Can you work these out from the drawing? Everything is in mm from the part's minimum corner. A direction names the side the tool comes from. Give positions to 0.01 mm unless a question says otherwise; leave off trailing zeros. Loops run counter-clockwise (first coordinate to the right, second up) from the corner with the lowest first, then second, coordinate; pieces in that order, holes last. Notation, with made-up numbers: (69, 71) - (128, 71) arc R20 cw to (128, 102) - close; hole circle Ø3 at (7.25, 51.5). An arc over 180 degrees is marked (long way). One line per item, written item: value. Start each with the question number.
Q1. For the marked faces 5, 6 and 7, which set-ups out of +Z, -Z, +X, -X, +Y, -Y let a thin tool reach every point of the face, with its end or its side?
Q2. If I drill on line 1 (Z direction, x = 33, y = 20); line 2 (Z direction, x = 6.5, y = 22.5); line 3 (X direction, y = 30, z = 86), over which ranges is the centre line in solid material (lowest first)? Write a range as from..to.
Q3. I want a section at D-D (y = 36). Please give me the cut outline in (x, z), then the cut area to 3 significant figures.
Q4. I want a section at B-B (y = 11.5). Please give me the cut outline in (x, z).
Q5. If we mould it in two halves opening along Z, with no side actions, what happens to the marked faces 1, 2, 3 and 4? For each: released by +Z, released by -Z, zero draft, split by the parting line, or undercut.
Q6. I'm going to push flat-ended pins straight in: P1, Ø23, axis at y = 20, z = 20, coming from the +X side; P2, Ø1.5, axis at x = 30.5, y = 35.5, coming from the +Z side; P3, Ø16, axis at y = 20, z = 100, coming from the +X side; P4, Ø10, axis at x = 17.5, y = 17.5, coming from the -Z side. Where does each tip first touch, or does it pass through?
Q7. I want a section at C-C (x = 8). Count the separate pieces of the cut face and the enclosed holes in it, then the cut area to 3 significant figures.
Q8. I want a section at A-A (z = 35.5). Please give me the cut outline in (x, y).
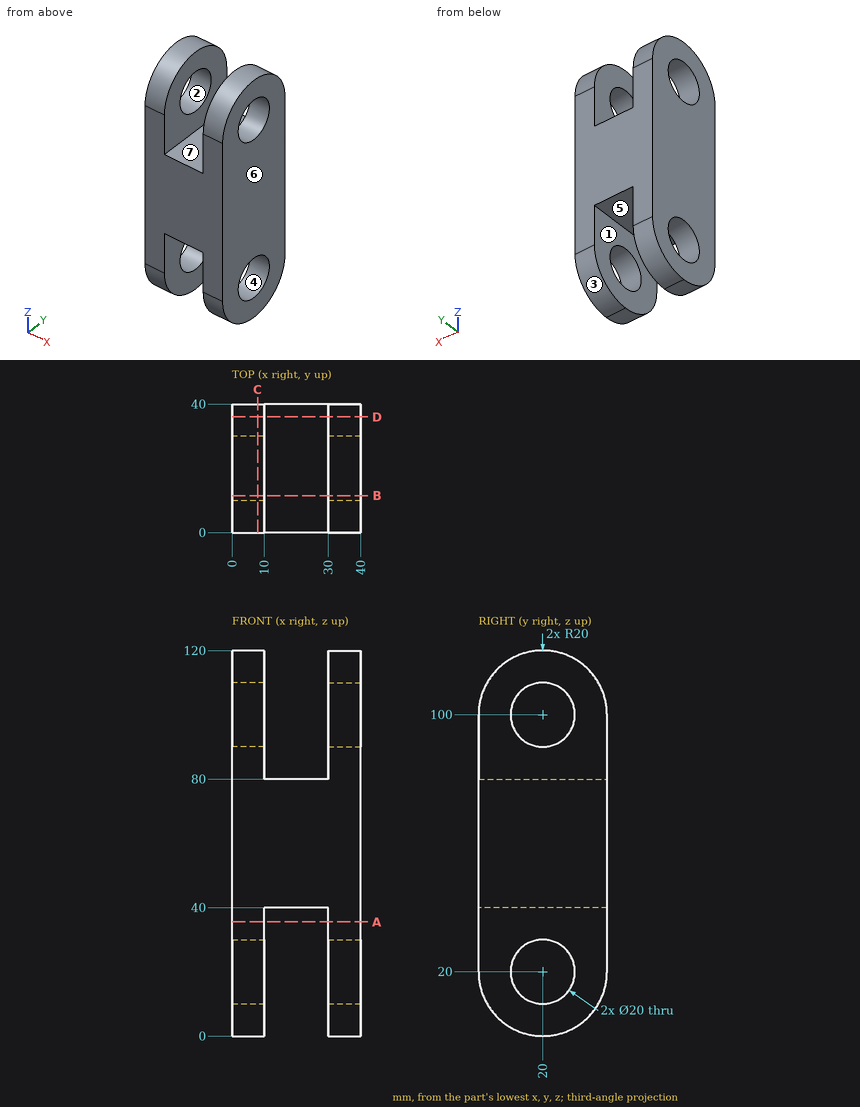
Worked answers:
1. face 5: -Z, +Y, -Y
1. face 6: +Z, -Z, +X, +Y, -Y
1. face 7: +Z, +Y, -Y
2. line 1: z = 0..10, 30..90, 110..120
2. line 2: z = 0.16..10.32, 29.68..90.32, 109.68..119.84
2. line 3: x = 0..10, 30..40
3. outline: (0, 8) - (10, 8) - (10, 40) - (30, 40) - (30, 8) - (40, 8) - (40, 112) - (30, 112) - (30, 80) - (10, 80) - (10, 112) - (0, 112) - close
3. area: 2,880 mm²
4. outline: (0, 1.9) - (10, 1.9) - (10, 14.73) - (0, 14.73) - close; (0, 25.27) - (10, 25.27) - (10, 40) - (30, 40) - (30, 25.27) - (40, 25.27) - (40, 94.73) - (30, 94.73) - (30, 80) - (10, 80) - (10, 94.73) - (0, 94.73) - close; (0, 105.27) - (10, 105.27) - (10, 118.1) - (0, 118.1) - close; (30, 1.9) - (40, 1.9) - (40, 14.73) - (30, 14.73) - close; (30, 105.27) - (40, 105.27) - (40, 118.1) - (30, 118.1) - close
5. face 1: zero draft
5. face 2: undercut
5. face 3: released by -Z
5. face 4: undercut
6. P1: stops at x = 40
6. P2: stops at z = 113.51
6. P3: passes through
6. P4: stops at z = 40
7. separate pieces: 1
7. enclosed holes: 2
7. area: 3,830 mm²
8. outline: (0, 0) - (10, 0) - (10, 40) - (0, 40) - close; (30, 0) - (40, 0) - (40, 40) - (30, 40) - close
